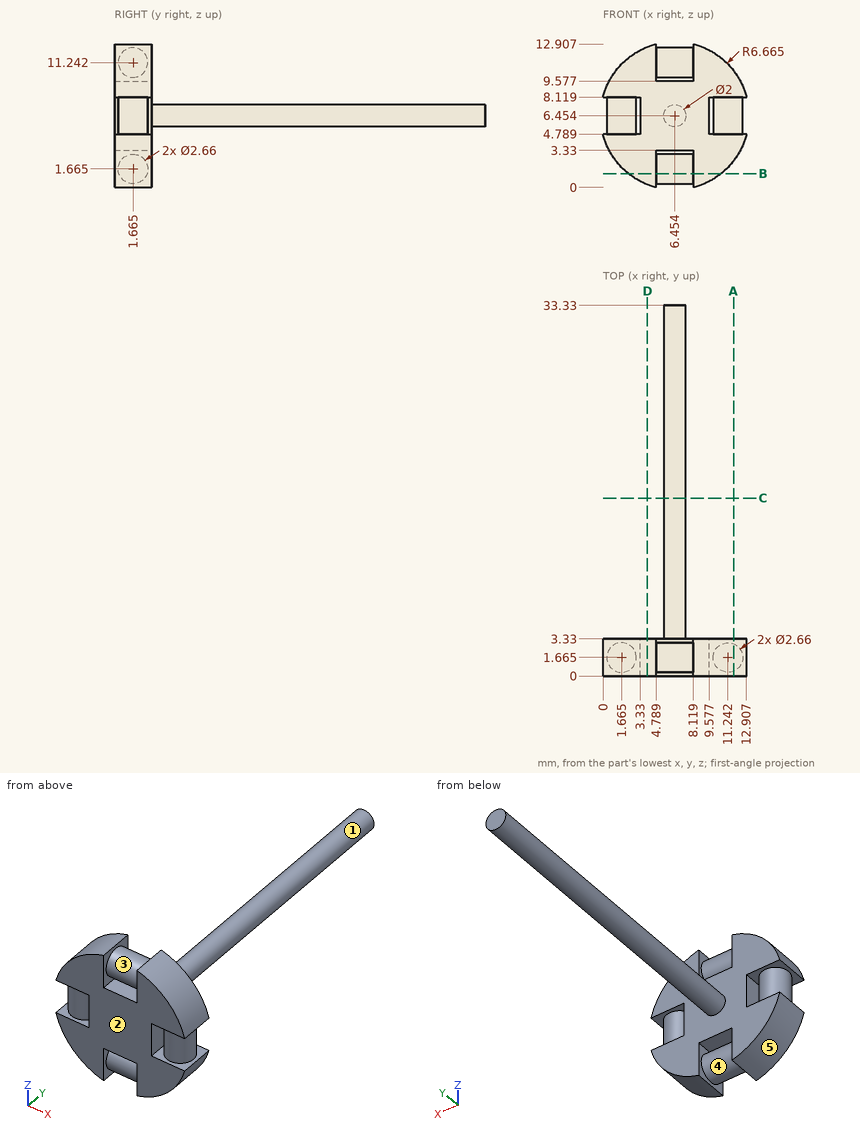
Here's the drawing with two shaded views (mm, measured from the low corner). I have some questions. A direction names the side the tool comes from. Coordinates: 2 decimals unless noted, no trailing zeros. Write each loop counter-clockwise with the first axis right and the second up, starting at its lowest first coordinate (ties: lowest second). Pieces come first, ordered by that corner, then holes. Notation, with made-up numbers: (-8, 39.5) -> (25, 39.5) arc R12 cw to (25, 59.5) -> close; hole circle Ø10 at (19, 41.25). An arc over 180 degrees is marked (long way). One line per question, with ' | ' between items. Start each with the question number.
1. If we section it at C-C (y = 16): Please give me the cut outline in (x, z).
2. Thinking about a two-plate mould opening in Z: for the marked faces 1, 2 and 3, which applies, pulls with the +Z half, pulls with the -Z half, needs draft (parallel to the pull), parting line crosses it, or undercut?
3. For the marked faces 4 and 5, which set-ups out of +Z, -Z, +X, -X, +Y, -Y let a thin tool reach every point of the face, with its end or its side?
4. Will these pins go through, and if not, where does the flat tip stop? P1, Ø3, axis at x = 7, z = 1.5, coming from the +Y side; P2, Ø3.5, axis at y = 1.5, z = 1.5, coming from the -X side; P3, Ø1.7, axis at x = 2, y = 2, coming from the +Z side.
5. Please list where these lines run through material, in increasing order: line 1 along Y through (x, z) = (10, 8.25); line 2 along Y through (x, z) = (11.25, 7) (1 decimal).
6. If we section it at B-B (z = 1.25): Please give me the cut outline in (x, y).
7. If we section it at D-D (x = 4): Please give me the cut outline in (y, z).
8. If we section it at A-A (x = 11.75): Please give me the cut outline in (y, z) (1 decimal).
Return value:
1) outline: circle Ø2 at (6.45, 6.45)
2) face 1: parting line crosses it | face 2: needs draft | face 3: undercut
3) face 4: none | face 5: -Z, -X, +Y, -Y
4) P1: stops at y = 3.33 | P2: stops at x = 0.61 | P3: stops at z = 12.06
5) line 1: y = 0 to 3.33 | line 2: y = 0.3 to 3
6) outline: (2.29, 0) -> (4.79, 0) -> (4.79, 0.4) -> (8.12, 0.4) -> (8.12, 0) -> (10.62, 0) -> (10.62, 3.33) -> (8.12, 3.33) -> (8.12, 2.93) -> (4.79, 2.93) -> (4.79, 3.33) -> (2.29, 3.33) -> close
7) outline: (0, 0.26) -> (3.33, 0.26) -> (3.33, 12.65) -> (0, 12.65) -> close
8) outline: (0, 2.4) -> (3.3, 2.4) -> (3.3, 4.8) -> (2.9, 4.8) -> (2.9, 8.1) -> (3.3, 8.1) -> (3.3, 10.5) -> (0, 10.5) -> (0, 8.1) -> (0.4, 8.1) -> (0.4, 4.8) -> (0, 4.8) -> close
